Here's how the part is built. I have some questions about the finished solid (model axes, mm). A direction names the side the tool comes from. Give positions to 0.01 mm unless a question says otherwise; leave off trailing zeros. Write each loop counter-clockwise with the first axis right and the second up, starting at its lowest first coordinate (ties: lowest second). Pieces come first, ordered by that corner, then holes. Notation, with made-up numbers: (13, -25) - (47, -25) arc R25 cw to (47, 10) - close; hole circle Ø6 at (71.5, 59.5). An arc over 180 degrees is marked (long way). Use a Markdown table: item, result.
```python
from build123d import *

# Parameters (mm, degrees)
SKETCH1_W           = 45
SKETCH1_H           = 27
SKETCH1_R           = 9.475
SKETCH1_R_2         = 1.24
BOSS_EXTRUDE1_DEPTH = 5
SKETCH1_3_W         = 49
SKETCH1_3_H         = 31
SKETCH1_3_W_2       = 45
SKETCH1_3_H_2       = 27
BOSS_EXTRUDE2_DEPTH = 11
SKETCH2_W           = 46.5
SKETCH2_H           = 1.75
SKETCH2_H_2         = 1.25
BOSS_EXTRUDE3_DEPTH = 34
BOSS_EXTRUDE4_REACH = 49.319
BOSS_EXTRUDE4_START = -2
SKETCH2_4_W         = 30
SKETCH2_4_H         = 2
SKETCH3_R           = 1.3
CUT_EXTRUDE2_DEPTH  = 62.769733689
SKETCH3_3_R         = 2.5
SKETCH3_3_R_2       = 1.3
CUT_EXTRUDE3_DEPTH  = 1.5
FILLET3_R           = 10
FILLET4_R           = 10
FILLET5_R           = 2
FILLET6_R           = 2
FILLET7_R           = 20
SKETCH4_R           = 11.475
SKETCH4_R_2         = 6.5
BOSS_EXTRUDE5_DEPTH = 0.5
FILLET8_R           = 0.5
CUT_EXTRUDE4_DEPTH  = 62.769733689
FILLET9_R           = 10


# Some blends are built 0.0001 mm under size
with BuildPart() as part:
    # Sketch1 → Boss-Extrude1 (new body)
    with BuildSketch(Plane(origin=(0, 0, 0), x_dir=(1, 0, 0), z_dir=(0, 1, 0))):
        Rectangle(SKETCH1_W, SKETCH1_H)
        with Locations(Location((2.75, 0, 0), (0, 0, 270))):
            Circle(SKETCH1_R, mode=Mode.SUBTRACT)
        with Locations(Location((-19.5, 9.5, 0), (0, 0, 270))):
            Circle(SKETCH1_R_2, mode=Mode.SUBTRACT)
        with Locations(Location((-19.5, -9.5, 0), (0, 0, 270))):
            Circle(SKETCH1_R_2, mode=Mode.SUBTRACT)
        with Locations(Location((19.5, -8.5, 0), (0, 0, 270))):
            Circle(SKETCH1_R_2, mode=Mode.SUBTRACT)
        with Locations(Location((19.5, 8.5, 0), (0, 0, 270))):
            Circle(SKETCH1_R_2, mode=Mode.SUBTRACT)
    extrude(amount=-BOSS_EXTRUDE1_DEPTH)

    # Sketch1<3> → Boss-Extrude2 (add)
    with BuildSketch(Plane(origin=(0, 0, 0), x_dir=(1, 0, 0), z_dir=(0, 1, 0))):
        Rectangle(SKETCH1_3_W, SKETCH1_3_H)
        Rectangle(SKETCH1_3_W_2, SKETCH1_3_H_2, mode=Mode.SUBTRACT)
    extrude(amount=-BOSS_EXTRUDE2_DEPTH)

    # Sketch2 → Boss-Extrude3 (add)
    with BuildSketch(Plane.XZ.offset(11)):
        with Locations((0, 16.375)):
            Rectangle(SKETCH2_W, SKETCH2_H)
        with Locations((0, 14.875)):
            Rectangle(SKETCH2_W, SKETCH2_H_2)
        with Locations((0, -14.875)):
            Rectangle(SKETCH2_W, SKETCH2_H_2)
        with Locations((0, -16.375)):
            Rectangle(SKETCH2_W, SKETCH2_H)
    extrude(amount=BOSS_EXTRUDE3_DEPTH)

    # Sketch2<4> → Boss-Extrude4 (add, up to next)
    with BuildSketch(Plane.XZ.offset(11).offset(BOSS_EXTRUDE4_START), mode=Mode.PRIVATE) as boss_extrude4_sk1:
        with Locations((0, 12.5)):
            Rectangle(SKETCH2_4_W, SKETCH2_4_H)
    boss_extrude4_tool1 = extrude(boss_extrude4_sk1.sketch, amount=-BOSS_EXTRUDE4_REACH, mode=Mode.PRIVATE) - part.part
    # Sketch2<4> → Boss-Extrude4 (add, up to next)
    with BuildSketch(Plane.XZ.offset(11).offset(BOSS_EXTRUDE4_START), mode=Mode.PRIVATE) as boss_extrude4_sk2:
        with Locations((0, -12.5)):
            Rectangle(SKETCH2_4_W, SKETCH2_4_H)
    boss_extrude4_tool2 = extrude(boss_extrude4_sk2.sketch, amount=-BOSS_EXTRUDE4_REACH, mode=Mode.PRIVATE) - part.part
    add(boss_extrude4_tool1.solids().sort_by_distance((0, -9, 12.5))[0])
    add(boss_extrude4_tool2.solids().sort_by_distance((0, -9, -12.5))[0])

    # Sketch3 → Cut-Extrude2 (cut, through all)
    with BuildSketch(Plane(origin=(0, 0, -17.25), x_dir=(-1, 0, 0), z_dir=(0, 0, -1))):
        with Locations((-15.75, -22)):
            Circle(SKETCH3_R)
        with Locations((8.25, -22)):
            Circle(SKETCH3_R)
        with Locations((8.25, -34)):
            Circle(SKETCH3_R)
        with Locations((-15.75, -34)):
            Circle(SKETCH3_R)
    extrude(amount=-CUT_EXTRUDE2_DEPTH, mode=Mode.SUBTRACT)

    # Sketch3<3> → Cut-Extrude3 (cut)
    # profile 1 of 4: a face of its own
    with BuildSketch(Plane(origin=(0, 0, -17.25), x_dir=(-1, 0, 0), z_dir=(0, 0, -1))):
        with Locations((-15.75, -22)):
            Circle(SKETCH3_3_R)
        with Locations((-15.75, -22)):
            Circle(SKETCH3_3_R_2, mode=Mode.SUBTRACT)
    # profile 2 of 4: a face of its own
    with BuildSketch(Plane(origin=(0, 0, -17.25), x_dir=(-1, 0, 0), z_dir=(0, 0, -1))):
        with Locations((-15.75, -34)):
            Circle(SKETCH3_3_R)
        with Locations((-15.75, -34)):
            Circle(SKETCH3_3_R_2, mode=Mode.SUBTRACT)
    # profile 3 of 4: a face of its own
    with BuildSketch(Plane(origin=(0, 0, -17.25), x_dir=(-1, 0, 0), z_dir=(0, 0, -1))):
        with Locations((8.25, -34)):
            Circle(SKETCH3_3_R)
        with Locations((8.25, -34)):
            Circle(SKETCH3_3_R_2, mode=Mode.SUBTRACT)
    # profile 4 of 4: a face of its own
    with BuildSketch(Plane(origin=(0, 0, -17.25), x_dir=(-1, 0, 0), z_dir=(0, 0, -1))):
        with Locations((8.25, -22)):
            Circle(SKETCH3_3_R)
        with Locations((8.25, -22)):
            Circle(SKETCH3_3_R_2, mode=Mode.SUBTRACT)
    cut_extrude3 = extrude(amount=-CUT_EXTRUDE3_DEPTH, mode=Mode.SUBTRACT)

    # Mirror1: Cut-Extrude3 across plane
    add(cut_extrude3.mirror(Plane.XY), mode=Mode.SUBTRACT)

    # Fillet3
    # the kernel refuses this fillet: 10 mm, written as the material it adds along each edge
    with BuildSketch(Plane(origin=(-23.25, -11, -15.5), x_dir=(0, 1, 0), z_dir=(1, 0, 0)), Plane(origin=(23.25, -11, 15.5), x_dir=(0, 1, 0), z_dir=(-1, 0, 0))) as fillet3_piece_1:
        with BuildLine():
            CenterArc((5.651327278, -10), FILLET3_R, 90, 34.41150867)
            Line((0, -1.75), (0, 0))
            Line((0, 0), (5.651327278, 0))
        make_face()
    extrude(amount=46.5)

    # Fillet4
    fillet4_edges = [part.edges().sort_by_distance(p)[0] for p in [
        (0, -11, 17.25),
        (0, -11, -17.25),
    ]]
    fillet(fillet4_edges, radius=FILLET4_R)

    # Fillet5
    # the kernel refuses this fillet: 2 mm, written as the material it adds along each edge
    with BuildSketch(Plane(origin=(-23.25, -11, 14.25), x_dir=(0, 0, -1), z_dir=(1, 0, 0))) as fillet5_piece_1_section:
        with BuildLine():
            CenterArc((FILLET5_R, -FILLET5_R), FILLET5_R, 90, 90)
            Line((0, -FILLET5_R), (0, 0))
            Line((0, 0), (FILLET5_R, 0))
        make_face()
    fillet5_piece_1 = extrude(amount=51.5, mode=Mode.PRIVATE)
    fillet5_piece_1 = split(fillet5_piece_1, bisect_by=Plane(origin=(-22.5, -11.128717382, 13.194770831), z_dir=(-1, 0, 0)), keep=Keep.TOP, mode=Mode.PRIVATE)
    add(fillet5_piece_1)
    with BuildSketch(Plane(origin=(-28.25, -11, 14.25), x_dir=(0, 0, -1), z_dir=(1, 0, 0))) as fillet5_piece_2_section:
        with BuildLine():
            CenterArc((FILLET5_R, -FILLET5_R), FILLET5_R, 90, 90)
            Line((0, -FILLET5_R), (0, 0))
            Line((0, 0), (FILLET5_R, 0))
        make_face()
    fillet5_piece_2 = extrude(amount=51.5, mode=Mode.PRIVATE)
    fillet5_piece_2 = split(fillet5_piece_2, bisect_by=Plane(origin=(0, -11.527561527, 13.5), z_dir=(0, 0, 1)), keep=Keep.TOP, mode=Mode.PRIVATE)
    fillet5_piece_2 = split(fillet5_piece_2, bisect_by=Plane(origin=(-22.5, -11.527561527, 13.95791508), z_dir=(1, 0, 0)), keep=Keep.TOP, mode=Mode.PRIVATE)
    add(fillet5_piece_2)
    with BuildSketch(Plane(origin=(-28.25, -11, 14.25), x_dir=(0, 0, -1), z_dir=(1, 0, 0))) as fillet5_piece_3_section:
        with BuildLine():
            CenterArc((FILLET5_R, -FILLET5_R), FILLET5_R, 90, 90)
            Line((0, -FILLET5_R), (0, 0))
            Line((0, 0), (FILLET5_R, 0))
        make_face()
    fillet5_piece_3 = extrude(amount=51.5, mode=Mode.PRIVATE)
    fillet5_piece_3 = split(fillet5_piece_3, bisect_by=Plane(origin=(22.5, -11.128717382, 13.194770831), z_dir=(1, 0, 0)), keep=Keep.TOP, mode=Mode.PRIVATE)
    add(fillet5_piece_3)
    with BuildSketch(Plane(origin=(23.25, -11, -14.25), x_dir=(0, 0, 1), z_dir=(-1, 0, 0))) as fillet5_piece_4_section:
        with BuildLine():
            CenterArc((FILLET5_R, -FILLET5_R), FILLET5_R, 90, 90)
            Line((0, -FILLET5_R), (0, 0))
            Line((0, 0), (FILLET5_R, 0))
        make_face()
    fillet5_piece_4 = extrude(amount=51.5, mode=Mode.PRIVATE)
    fillet5_piece_4 = split(fillet5_piece_4, bisect_by=Plane(origin=(22.5, -11.128717382, -13.194770831), z_dir=(1, 0, 0)), keep=Keep.TOP, mode=Mode.PRIVATE)
    add(fillet5_piece_4)
    with BuildSketch(Plane(origin=(28.25, -11, -14.25), x_dir=(0, 0, 1), z_dir=(-1, 0, 0))) as fillet5_piece_5_section:
        with BuildLine():
            CenterArc((FILLET5_R, -FILLET5_R), FILLET5_R, 90, 90)
            Line((0, -FILLET5_R), (0, 0))
            Line((0, 0), (FILLET5_R, 0))
        make_face()
    fillet5_piece_5 = extrude(amount=51.5, mode=Mode.PRIVATE)
    fillet5_piece_5 = split(fillet5_piece_5, bisect_by=Plane(origin=(22.5, -11.527561527, -13.95791508), z_dir=(-1, 0, 0)), keep=Keep.TOP, mode=Mode.PRIVATE)
    fillet5_piece_5 = split(fillet5_piece_5, bisect_by=Plane(origin=(0, -11.527561527, -13.5), z_dir=(0, 0, -1)), keep=Keep.TOP, mode=Mode.PRIVATE)
    add(fillet5_piece_5)
    with BuildSketch(Plane(origin=(28.25, -11, -14.25), x_dir=(0, 0, 1), z_dir=(-1, 0, 0))) as fillet5_piece_6_section:
        with BuildLine():
            CenterArc((FILLET5_R, -FILLET5_R), FILLET5_R, 90, 90)
            Line((0, -FILLET5_R), (0, 0))
            Line((0, 0), (FILLET5_R, 0))
        make_face()
    fillet5_piece_6 = extrude(amount=51.5, mode=Mode.PRIVATE)
    fillet5_piece_6 = split(fillet5_piece_6, bisect_by=Plane(origin=(-22.5, -11.128717382, -13.194770831), z_dir=(-1, 0, 0)), keep=Keep.TOP, mode=Mode.PRIVATE)
    add(fillet5_piece_6)

    # Fillet6
    fillet6_edges = [part.edges().sort_by_distance(p)[0] for p in [
        (0, -11.4387505, 13.5),
        (0, -11.4387505, -13.5),
    ]]
    fillet(fillet6_edges, radius=FILLET6_R)

    # Fillet7
    fillet7_edges = [part.edges().sort_by_distance(p)[0] for p in [
        (-23.25, -45, 15.75),
        (23.25, -45, 15.75),
        (23.25, -45, -15.75),
        (-23.25, -45, -15.75),
    ]]
    fillet(fillet7_edges, radius=FILLET7_R)

    # Sketch4 → Boss-Extrude5 (add)
    with BuildSketch(Plane(origin=(0, 0, 0), x_dir=(1, 0, 0), z_dir=(0, 1, 0))):
        with Locations(Location((2.75, 0, 0), (0, 0, 270))):
            Circle(SKETCH4_R)
        with Locations(Location((2.75, 0, 0), (0, 0, 270))):
            Circle(SKETCH4_R_2, mode=Mode.SUBTRACT)
    extrude(amount=BOSS_EXTRUDE5_DEPTH)

    # Fillet8
    fillet8_edges = [part.edges().sort_by_distance(p)[0] for p in [
        (2.75, 0.5, -11.475),
        (2.75, 0.5, -6.5),
    ]]
    fillet(fillet8_edges, radius=FILLET8_R - 0.0001)  # a hair under: the kernel refuses the full size

    # Sketch5 → Cut-Extrude4 (cut, through all)
    with BuildSketch(Plane(origin=(0, 0, -17.25), x_dir=(-1, 0, 0), z_dir=(0, 0, -1))):
        with BuildLine():
            Line((-11.967797887, -43), (11.967797887, -43))
            ThreePointArc((11.967797887, -43), (7.722135955, -44.49358869), (3.25, -45))
            Line((3.25, -45), (-3.25, -45))
            ThreePointArc((-3.25, -45), (-7.722135955, -44.49358869), (-11.967797887, -43))
        make_face()
    extrude(amount=-CUT_EXTRUDE4_DEPTH, mode=Mode.SUBTRACT)

    # Fillet9
    fillet9_edges = [part.edges().sort_by_distance(p)[0] for p in [
        (11.967797887, -43, -15.75),
        (-11.967797887, -43, 15.75),
        (11.967797887, -43, 15.75),
        (-11.967797887, -43, -15.75),
    ]]
    fillet(fillet9_edges, radius=FILLET9_R)


solid = part.part
```
Item 1: I need wall thicknesses on line 1 along Y through (x, z) = (-8.25, -16.3); line 2 along Y through (x, z) = (-8.25, -15.2); line 3 along Z through (x, y) = (-13, -36). Which ranges of each line are inside material? Lowest first, please. Write a range as [from, to].
Values:
| item | result |
|---|---|
| line 1 | y = [-43, -36.5], [-31.5, -24.5], [-19.5, -9.27] |
| line 2 | y = [-43, -35.3], [-32.7, -23.3], [-20.7, 0] |
| line 3 | z = [-17.25, -14.25], [14.25, 17.25] |
Item 2: If we section it at B-B, the plane y = -3.5: Write out the boundary of the cut face in (x, z) (3 decimals).
Values:
| item | result |
|---|---|
| outline | (-24.5, -15.5) - (24.5, -15.5) - (24.5, 15.5) - (-24.5, 15.5) - close; hole circle Ø2.48 at (-19.5, -9.5); hole circle Ø2.48 at (-19.5, 9.5); hole circle Ø18.95 at (2.75, 0); hole circle Ø2.48 at (19.5, -8.5); hole circle Ø2.48 at (19.5, 8.5) |
Item 3: Thinking about a two-plate mould opening in X: for faces 1 (the cylindrical face through (-9.59, -31.89, 16.51)), 2 (the cylindrical face through (21.08, -34.06, -15.73)), 3 (the flat face through (0, -43, -16)), which applies, +X half, -X half, draft (parallel to the pull), parting line (faces both ways), or undercut?
Values:
| item | result |
|---|---|
| face 1 | undercut |
| face 2 | +X half |
| face 3 | draft |
Item 4: For faces 4 (the flat face through (-9.3, -35.1, 15.75)), 5 (the flat face through (15, -7, -13)), 6 (the flat face through (-24, -11, 0)), 7 (the flat face through (14.7, -35.1, -15.75)), 8 (the cylindrical face through (-21.08, -34.06, -15.77)), which set-ups out of +Z, -Z, +X, -X, +Y, -Y let a thin tool reach every point of the face, with its end or its side?
Values:
| item | result |
|---|---|
| face 4 | +Z |
| face 5 | -Y |
| face 6 | -X, -Y |
| face 7 | -Z |
| face 8 | +Z, -Z, -X, -Y |
Item 5: If we section it at D-D, the plane x = 19.5: Write out the boundary of the cut face in (y, z) (3 decimals).
Values:
| item | result |
|---|---|
| outline | (-36.659, -17.25) - (-13.53, -17.25) arc R10 ccw to (-9.439, -16.375) arc R10 cw to (-5.349, -15.5) - (0, -15.5) - (0, -9.74) - (-5, -9.74) - (-5, -13.5) - (-10.668, -13.5) arc R2 ccw to (-11.834, -13.875) arc R2 cw to (-13, -14.25) - (-36.659, -14.25) - close; (-36.659, 14.25) - (-13, 14.25) arc R2 cw to (-11.834, 13.875) arc R2 ccw to (-10.668, 13.5) - (-5, 13.5) - (-5, 9.74) - (0, 9.74) - (0, 15.5) - (-5.349, 15.5) arc R10 cw to (-9.439, 16.375) arc R10 ccw to (-13.53, 17.25) - (-36.659, 17.25) - close; (-5, -7.26) - (0, -7.26) - (0, 7.26) - (-5, 7.26) - close |
Item 6: Will these pins go through, and if not, where does the flat tip stop? pin 1 Ø4.5 at (x, y) = (-6, -6.5) entering from -Z; pin 2 Ø2.5 at (x, y) = (16.5, -33.5) entering from +Z; pin 3 Ø5.5 at (x, y) = (-1.5, -6.5) entering from -Z.
Values:
| item | result |
|---|---|
| pin 1 | stops at z = -16.1 |
| pin 2 | stops at z = 15.75 |
| pin 3 | stops at z = -16.29 |
Item 7: If we section it at A-A, the plane y = -15.5: Write out the boundary of the cut face in (x, z), plus the area to 3 significant figures.
Values:
| item | result |
|---|---|
| outline | (-23.25, -17.25) - (23.25, -17.25) - (23.25, -14.25) - (-23.25, -14.25) - close; (-23.25, 14.25) - (23.25, 14.25) - (23.25, 17.25) - (-23.25, 17.25) - close |
| area | 279 mm2 |
